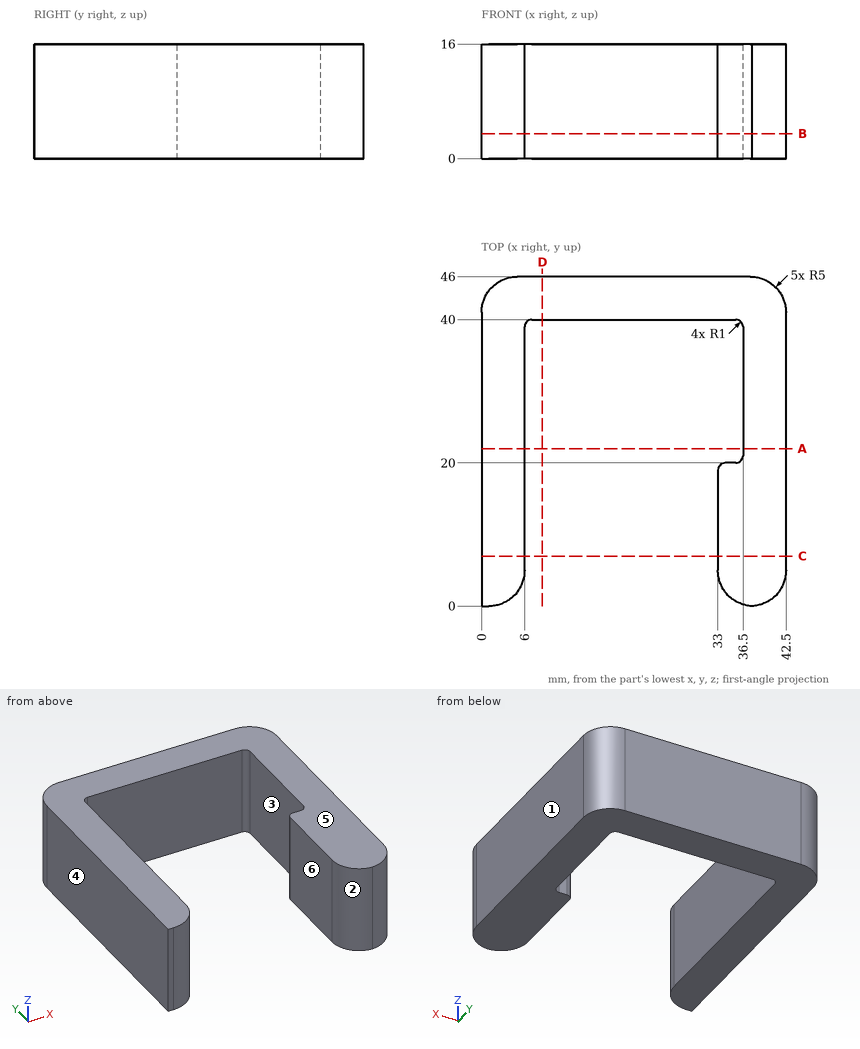
Drawing for the job (mm, zero at the part's lowest x, y, z). A direction names the side the tool comes from. Round coordinates to 2 decimals unless told otherwise and drop trailing zeros. Order: outer loops, then holes, each group sorted by start corner. A loop starts at its lowest first (then second) coordinate and runs counter-clockwise, first axis right, second up. Notation, with made-up numbers: (41, 86.5) -> (88, 86.5) arc R32 ccw to (88, 118.5) -> close; hole circle Ø7 at (82.25, -25.75). An arc over 180 degrees is marked (long way). Write item = value, one per line. Start each with the question number.
(1) Which spindle directions (+Z, -Z, +X, -X, +Y, -Y) get a long thin tool onto all of the face, cutting with end or side? Do the marked faces 1, 2 and 3. Say none if no direction does.
(2) Cut at A-A, the plane y = 22. List the corners of the cut face in (x, z), then the cut area to 3 significant figures.
(3) Pin check, flat tip, straight feed: P1, Ø1, axis at x = 15.5, z = 5, coming from the -Y side. Stop position of the tip, or through.
(4) Cut at C-C, the plane y = 7. List the corners of the cut face in (x, z), then the cut area to 3 significant figures.
(5) Cut at B-B, the plane z = 3.5. List the corners of the cut face in (x, y), then the cut area to 3 significant figures.
(6) Pull direction X, two halves, no side cores. Call the marked faces 4, 5 and 6: released by +X, released by -X, zero draft, split by the parting line, or undercut.
(7) Cut at D-D, the plane x = 8.5. List the corners of the cut face in (y, z), then the cut area to 3 significant figures.
(8) Probe line 1 (X direction, y = 39, z = 14.5); line 2 (X direction, y = 5.5, z = 6.5); line 3 (Y direction, x = 35, z = 1.25). List the from-to ranges inside material, lowest first. Write a range as [from, to].
Model answer:
q1.face_1 = +Z, -Z, +X, +Y, -Y
q1.face_2 = +Z, -Z, -Y
q1.face_3 = +Z, -Z
q2.outline = (0, 0) -> (6, 0) -> (6, 16) -> (0, 16) -> close; (36.5, 0) -> (42.5, 0) -> (42.5, 16) -> (36.5, 16) -> close
q2.area = 192 mm2
q3.P1 = 40
q4.outline = (0, 0) -> (6, 0) -> (6, 16) -> (0, 16) -> close; (33, 0) -> (42.5, 0) -> (42.5, 16) -> (33, 16) -> close
q4.area = 248 mm2
q5.outline = (0, 0) -> (1, 0) arc R5 ccw to (6, 5) -> (6, 39) arc R1 cw to (7, 40) -> (35.5, 40) arc R1 cw to (36.5, 39) -> (36.5, 21) arc R1 cw to (35.5, 20) -> (34, 20) arc R1 ccw to (33, 19) -> (33, 5) arc R5 ccw to (37.75, 0.01) arc R5 ccw to (42.5, 5) -> (42.5, 41) arc R5 ccw to (37.5, 46) -> (5, 46) arc R5 ccw to (0, 41) -> close
q5.area = 779 mm2
q6.face_4 = released by -X
q6.face_5 = zero draft
q6.face_6 = undercut
q7.outline = (40, 0) -> (46, 0) -> (46, 16) -> (40, 16) -> close
q7.area = 96.0 mm2
q8.line_1 = [0, 6], [36.5, 42.5]
q8.line_2 = [0, 6], [33, 42.5]
q8.line_3 = [1, 20], [40, 46]
